Job drawing, mm, ordinate dimensions from the low corner. One solid piece. Round coordinates to 2 decimals unless told otherwise and drop trailing zeros. Order: outer loops, then holes, each group sorted by start corner. A loop starts at its lowest first (then second) coordinate and runs counter-clockwise, first axis right, second up. Notation, with made-up numbers: (18.5, 6.25) -> (24.5, 6.25) arc R6 ccw to (24.5, 17.25) -> close; hole circle Ø4 at (6, 53.5). An arc over 180 degrees is marked (long way). Return JSON: item names as keys, results as strings. Group by question number.
Q1. Mould opens along X. For the marked faces 1, 2 and 3 say: +X half, -X half, draft (parallel to the pull), parting line (faces both ways), or undercut.
Q2. Flat gauge pins, fed straight in: pin 1 (1.5 mm diameter, centred on x = 38, z = 21, fed in from +Y); pin 2 (6.5 mm diameter, centred on y = 22, z = 15, fed in from +X); pin 3 (1.5 mm diameter, centred on x = 26.5, y = 39, fed in from +Z); pin 4 (2 mm diameter, centred on y = 32, z = 25, fed in from +X). Where does each tip first touch, or does it go through?
Q3. Cut at C-C (x = 20). Write the cut outline in (y, z), then the cut area to 3 significant figures.
Q4. Cut at A-A (z = 25). Write the cut outline in (x, y).
Q5. Probe line 1 along Z through (x, y) = (39.05, 32); line 2 along X through (y, z) = (1.9, 5); line 3 along X through (y, z) = (24.5, 4). List the from-to ranges inside material, lowest first.
Q6. Cut at D-D (z = 15). Write the cut outline in (x, y).
Q7. Cut at B-B (y = 12). Write the cut outline in (x, z).
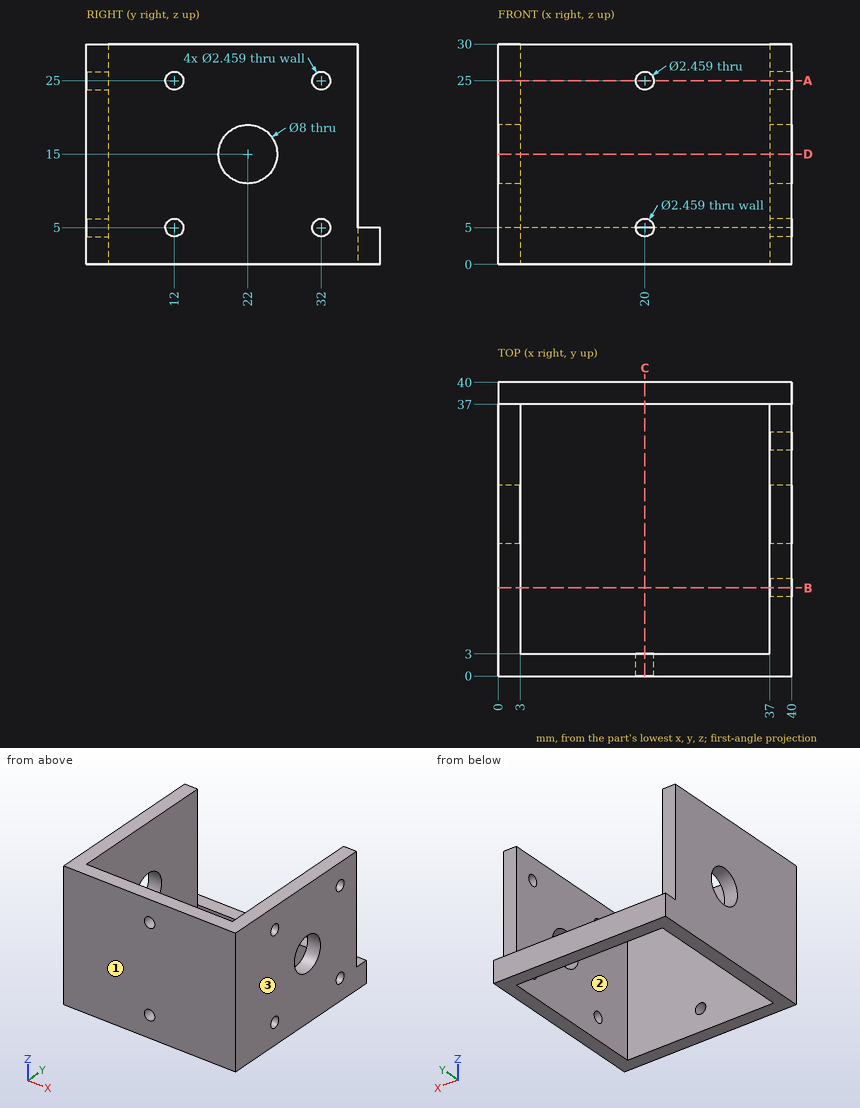
Solution:
{
 "1": {"face 1": "draft", "face 2": "undercut", "face 3": "+X half"},
 "2": {"pin 1": "stops at y = 37", "pin 2": "passes through", "pin 3": "stops at z = 5", "pin 4": "stops at x = 3"},
 "3": {"outline": "(0, 0) -> (3, 0) -> (3, 3.77) -> (0, 3.77) -> close; (0, 6.23) -> (3, 6.23) -> (3, 23.77) -> (0, 23.77) -> close; (0, 26.23) -> (3, 26.23) -> (3, 30) -> (0, 30) -> close; (37, 0) -> (40, 0) -> (40, 5) -> (37, 5) -> close", "area": "90.2 mm²"},
 "4": {"outline": "(0, 0) -> (18.77, 0) -> (18.77, 3) -> (3, 3) -> (3, 37) -> (0, 37) -> close; (21.23, 0) -> (40, 0) -> (40, 10.77) -> (37, 10.77) -> (37, 3) -> (21.23, 3) -> close; (37, 13.23) -> (40, 13.23) -> (40, 30.77) -> (37, 30.77) -> close; (37, 33.23) -> (40, 33.23) -> (40, 37) -> (37, 37) -> close"},
 "5": {"line 1": "z = 0 to 3.77, 6.23 to 23.77, 26.23 to 30", "line 2": "x = 0 to 18.77, 21.23 to 40", "line 3": "x = 0 to 3, 37 to 40"},
 "6": {"outline": "(0, 0) -> (40, 0) -> (40, 18) -> (37, 18) -> (37, 3) -> (3, 3) -> (3, 18) -> (0, 18) -> close; (0, 26) -> (3, 26) -> (3, 37) -> (0, 37) -> close; (37, 26) -> (40, 26) -> (40, 37) -> (37, 37) -> close"},
 "7": {"outline": "(0, 0) -> (3, 0) -> (3, 30) -> (0, 30) -> close; (37, 0) -> (40, 0) -> (40, 3.77) -> (37, 3.77) -> close; (37, 6.23) -> (40, 6.23) -> (40, 23.77) -> (37, 23.77) -> close; (37, 26.23) -> (40, 26.23) -> (40, 30) -> (37, 30) -> close"}
}
